The listing builds one solid part. Answer for the finished solid, in the listing's coordinates (mm). Face numbers are marked on the shaded views. A direction names the side the tool comes from. Round coordinates to 2 decimals unless told otherwise and drop trailing zeros. Write each loop counter-clockwise with the first axis right and the second up, starting at its lowest first coordinate (ties: lowest second). Pieces come first, ordered by that corner, then holes.
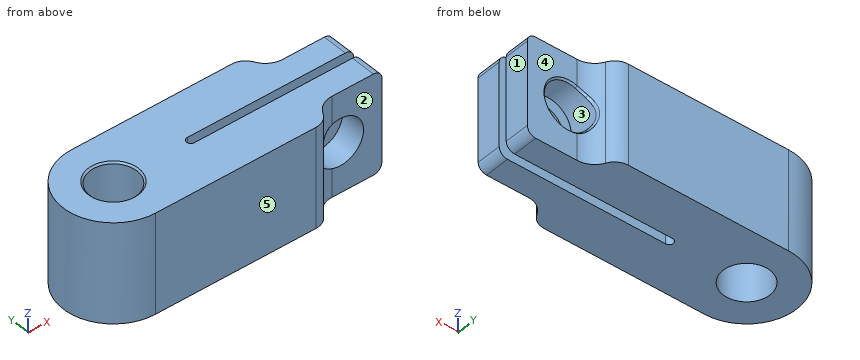
Autodesk Inventor part; units mm, degrees
ref_plane "YZ Plane" through (0, 0, 0) normal (1, 0, 0) x (0, 1, 0)
ref_plane "XZ Plane" through (0, 0, 0) normal (0, 1, 0) x (-1, 0, 0)
ref_plane "XY Plane" through (0, 0, 0) normal (0, 0, 1) x (1, 0, 0)
sketch "Sketch1" plane through (0, 0, 0) normal (0, 0, 1) x (1, 0, 0)
  line L0 (0, 0) -> (0, 0.56) construction
  line L1 (0, 0) -> (-1.0158, 0) construction
  line L2 (-4.65, 3) -> (5.75, 3)
  line L3 (5.75, -3) -> (-4.65, -3)
  line L4 (10, 0.25) -> (0, 0.25)
  line L5 (10, -0.25) -> (0, -0.25)
  arc A0 (0, 0.25) -> (0, -0.25) centre (0, 0) ccw
  line L6 (10, 1.75) -> (7, 1.75)
  line L7 (10, -1.75) -> (7, -1.75)
  arc A1 (-4.65, 3) -> (-4.65, -3) centre (-4.65, 0) ccw
  circle A2 centre (-4.65, 0) radius 1.4
  line L8 (10, 1.75) -> (10, 0.25)
  line L9 (10, -0.25) -> (10, -1.75)
  arc A3 (5.75, 3) -> (7, 1.75) centre (7, 3) ccw
  arc A4 (7, -1.75) -> (5.75, -3) centre (7, -3) ccw
  dimension "d2" = 0.5
  dimension "d5" = 2.8
  dimension "d6" = 6
  dimension "d8" = 10
  dimension "d9" = 1.5
  dimension "d10" = 3
  dimension "d12" = 3
extrude "Extrusion1" add sketch "Sketch1" along normal blind 6
sketch "Sketch2" plane through (7, 1.75, 0) normal (0, 1, 0) x (1, 0, 0)
  circle A0 centre (0.5, -3.0099) radius 1.4
  line L0 (3, 0) -> (3, -6)
  point P0 (-7, 0)
  dimension "d15" = 2.8
  dimension "d16" = 2.5
extrude "Extrusion2" cut sketch "Sketch2" along normal through all both and the other way through all
fillet "Fillet1" radius 0.5 1 edges at (10, 1, 6)
fillet "Fillet2" radius 0.5 1 edges at (10, -1, 6)
fillet "Fillet3" radius 0.5 1 edges at (10, 1, 0)
fillet "Fillet4" radius 0.5 1 edges at (10, -1, 0)
fillet "Fillet5" radius 1 1 edges at (5.75, 3, 3)
fillet "Fillet6" radius 1 1 edges at (5.75, -3, 3)
chamfer "Chamfer1" distance 0.1 angle 45 1 edges at (-6.05, 0, 6)
chamfer "Chamfer2" distance 0.1 angle 45 3 edges at (6.1, 2.1325, 3.0079) (8.2937, 1.75, 1.8567) (8.2937, 1.75, 4.1632)
equation "\"d17\" = d15"
properties part number "StringClamp"
1. Given pin 1 (1.7 mm diameter, centred on x = 7.5, z = 3.01, fed in from +Y); pin 2 (0.9 mm diameter, centred on x = 8, z = 4.5, fed in from -Y); pin 3 (3.5 mm diameter, centred on x = 8, z = 1.5, fed in from +Y), each flat-ended and moving along its own axis, determine where each tip first touches the part or whether it passes through.
Geometry says:
pin 1: passes through
pin 2: stops at y = -1.75
pin 3: stops at y = 2
2. Straight lines are drawn through the part: line 1 along Y through (x, z) = (3.5, 2.75); line 2 along Y through (x, z) = (-4.65, 3.45); line 3 along X through (y, z) = (-0.85, 2). For each, find the intervals that lie inside material, in ascending order.
Geometry says:
line 1: y = -3 to -0.25, 0.25 to 3
line 2: y = -3 to -1.4, 1.4 to 3
line 3: x = -7.53 to -5.76, -3.54 to 6.53, 8.47 to 10
3. Section B-B on x = 1 is taken. Determine the outline of the cut face in (y, z).
Geometry says:
outline: (-3, 0) - (-0.25, 0) - (-0.25, 6) - (-3, 6) - close; (0.25, 0) - (3, 0) - (3, 6) - (0.25, 6) - close
4. Section C-C on x = 7.5 is taken. Determine the outline of the cut face in (y, z), plus the area to 3 significant figures.
Geometry says:
outline: (-1.75, 0) - (-0.25, 0) - (-0.25, 1.61) - (-1.75, 1.61) - close; (-1.75, 4.41) - (-0.25, 4.41) - (-0.25, 6) - (-1.75, 6) - close; (0.25, 0) - (1.75, 0) - (1.75, 1.51) - (1.65, 1.61) - (0.25, 1.61) - close; (0.25, 4.41) - (1.65, 4.41) - (1.75, 4.51) - (1.75, 6) - (0.25, 6) - close
area: 9.59 mm2
5. Section A-A on y = 0 is taken. Determine the outline of the cut face in (x, z).
Geometry says:
outline: (-7.65, 0) - (-6.05, 0) - (-6.05, 5.9) - (-6.15, 6) - (-7.65, 6) - close; (-3.25, 0) - (-0.25, 0) - (-0.25, 6) - (-3.15, 6) - (-3.25, 5.9) - close
6. A tool of negligible diameter and unlimited length cuts with its end or side. For the marked faces 4 and 5, from which of +Z, -Z, +X, -X, +Y, -Y can it reach the whole face along a straight path? Write none if from no direction.
Geometry says:
face 4: +Z, -Z, +X, +Y
face 5: +Z, -Z, +X, -X, -Y
7. For a pull along X with two mould halves and no side action, classify the marked faces 1, 2 and 3 as released by +X, released by -X, zero draft, split by the parting line, or undercut.
Geometry says:
face 1: released by +X
face 2: zero draft
face 3: undercut
8. Section D-D on z = 3.5 is taken. Give the number of separate pieces and of enclosed holes in the cut face, plus the area to 3 significant figures.
Geometry says:
separate pieces: 3
enclosed holes: 1
area: 72.6 mm2
